from build123d import *

# Parameters (mm, degrees)
F0_R     = 33.082468
F1_DEPTH = 25
F2_R     = 15.300047
F3_DEPTH = 25
F4_SIZE  = 5
F5_R     = 15.3009
F6_DEPTH = 25


with BuildPart() as f1:
    # F0 (on Top) → F1 (new body)
    with BuildSketch(Plane.XY):
        Circle(F0_R)
    extrude(amount=F1_DEPTH)

    # F2 (on face) → F3 (join)
    with BuildSketch(Plane.XY.offset(25)):
        Circle(F2_R)
    extrude(amount=F3_DEPTH)

    # F4
    f4_edges = [f1.edges().sort_by_distance(p)[0] for p in [
        (-15.300047, 0, 50),
    ]]
    chamfer(f4_edges, length=F4_SIZE)

    # F5 (on face) → F6 (join)
    with BuildSketch(Plane(origin=(0, 0, 0), x_dir=(1, 0, 0), z_dir=(0, 0, -1))):
        Circle(F5_R)
    extrude(amount=F6_DEPTH)


solid = f1.part
The model under review builds one solid part; all positions refer to its coordinate system, in mm. A direction names the side the tool comes from. Round coordinates to 2 decimals unless told otherwise and drop trailing zeros. Write each loop counter-clockwise with the first axis right and the second up, starting at its lowest first coordinate (ties: lowest second). Pieces come first, ordered by that corner, then holes. Notation, with made-up numbers: (0, 53.25) - (25, 53.25) arc R16 cw to (25, 61.25) - close; hole circle Ø8 at (21, 24.25). An arc over 180 degrees is marked (long way). One line per item, written item: value. Start each with the question number.
1. Machinability: for faces 1 (the face through (14, -7, 25)), 2 (the face through (-3.317, 14.937, -12.325)), 3 (the face through (0, 0, 50)), which of the approach directions +Z, -Z, +X, -X, +Y, -Y give a long, thin tool a straight path to every point of the face, cutting with its end or side? Answer none if there is none.
2. To check wall thickness, follow L1, parallel to Z at x = -17.5, y = -7.5; L2, parallel to Y at x = -0.5, z = -8.5; L3, parallel to X at y = 7, z = -21. State the ranges of each line that lie inside material, in increasing order. Write a range as from..to.
3. Consider section C-C on z = 33. Write out the cut boundary in (x, y).
4. Clearance check with flat-ended pins moving along their axes: P1, Ø2, axis at x = -11, z = 39, coming from the +Y side; P2, Ø5, axis at x = -1.5, y = -26.5, coming from the -Z side; P3, Ø10, axis at y = -15.5, z = 36, coming from the +X side. State where each tip first meets the part, or that it passes through.
5. Consider section A-A on x = 0. Write out the cut boundary in (y, z), and give its area (3 significant figures).
Checks:
1. face 1: +Z
1. face 2: -Z
1. face 3: +Z, +X, -X, +Y, -Y
2. L1: z = 0..25
2. L2: y = -15.29..15.29
2. L3: x = -13.61..13.61
3. outline: circle Ø30.6 at (0, 0)
4. P1: stops at y = 11.58
4. P2: stops at z = 0
4. P3: stops at x = 11.13
5. outline: (-33.08, 0) - (-15.3, 0) - (-15.3, -25) - (15.3, -25) - (15.3, 0) - (33.08, 0) - (33.08, 25) - (15.3, 25) - (15.3, 45) - (10.3, 50) - (-10.3, 50) - (-15.3, 45) - (-15.3, 25) - (-33.08, 25) - close
5. area: 3,160 mm^2
